from build123d import *

# Parameters (mm, degrees)
F0_W     = 57.15
F0_H     = 38.1
F1_DEPTH = 38.1
F3_DEPTH = 12.7
F5_DEPTH = 12.7


with BuildPart() as f1:
    # F0 (on Front) → F1 (new body)
    with BuildSketch(Plane.XZ):
        with Locations((28.575, 19.05)):
            Rectangle(F0_W, F0_H)
    extrude(amount=-F1_DEPTH)

    # F2 (on face) → F3 (cut)
    with BuildSketch(Plane.XZ):
        Polygon((57.15, 38.1), (19.05, 38.1), (25.4, 0), (57.15, 0), align=None)
    extrude(amount=-F3_DEPTH, mode=Mode.SUBTRACT)

    # F4 (on face) → F5 (cut)
    with BuildSketch(Plane(origin=(0, 38.1, 0), x_dir=(-1, 0, 0), z_dir=(0, 1, 0))):
        Polygon((-25.4, 0), (-19.05, 38.1), (-57.15, 38.1), (-57.15, 0), align=None)
    extrude(amount=-F5_DEPTH, mode=Mode.SUBTRACT)


solid = f1.part
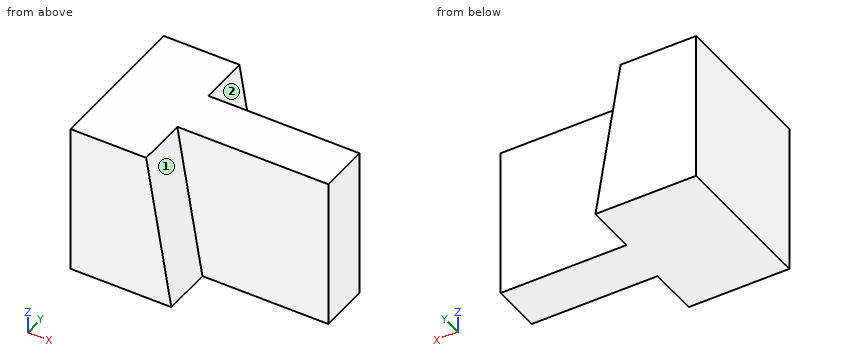
Geometry: final body of the model. Coordinates: model frame, mm. Face numbers are marked on the shaded views. A direction names the side the tool comes from. Coordinates: 2 decimals unless noted, no trailing zeros. Order: outer loops, then holes, each group sorted by start corner. A loop starts at its lowest first (then second) coordinate and runs counter-clockwise, first axis right, second up.
(1) Access query for the marked faces 1 and 2. Directions: +Z, -Z, +X, -X, +Y, -Y. A direction counts if a zero-diameter tool reaches every point of the face in a straight line with its end or side. Return the directions, or none.
(2) Section query C-C (y = 31). Return the cut outline in (x, z), plus the area to 3 significant figures.
(3) Section query B-B (z = 9). Return the cut outline in (x, y), plus the area to 3 significant figures.
(4) Section query A-A (x = 23.5). Return the cut outline in (y, z), plus the area to 3 significant figures.
(5) First-contact query: pin 1 (12 mm diameter, centred on x = 31, z = 8, fed in from +Y); pin 2 (19 mm diameter, centred on x = 44.5, z = 18.5, fed in from -Y). Flat tips, straight axial feed; report the tip coordinate or a pass-through.
(6) Material intervals for probe 1 along Y at (x, z) = (53.5, 17); probe 2 along X at (y, z) = (11.5, 28.5); probe 3 along X at (y, z) = (25.5, 5.5), sorted ascending.
(7) Section query D-D (x = 42.5). Return the cut outline in (y, z), plus the area to 3 significant figures.
Solution:
1. face 1: +Z, +X, -Y
1. face 2: +Z, +X, +Y
2. outline: (0, 0) - (25.4, 0) - (19.05, 38.1) - (0, 38.1) - close
2. area: 847 mm2
3. outline: (0, 0) - (23.9, 0) - (23.9, 12.7) - (57.15, 12.7) - (57.15, 25.4) - (23.9, 25.4) - (23.9, 38.1) - (0, 38.1) - close
3. area: 1,330 mm2
4. outline: (0, 0) - (38.1, 0) - (38.1, 11.4) - (25.4, 11.4) - (25.4, 38.1) - (12.7, 38.1) - (12.7, 11.4) - (0, 11.4) - close
4. area: 773 mm2
5. pin 1: stops at y = 25.4
5. pin 2: stops at y = 12.7
6. probe 1: y = 12.7 to 25.4
6. probe 2: x = 0 to 20.65
6. probe 3: x = 0 to 24.48
7. outline: (12.7, 0) - (25.4, 0) - (25.4, 38.1) - (12.7, 38.1) - close
7. area: 484 mm2
